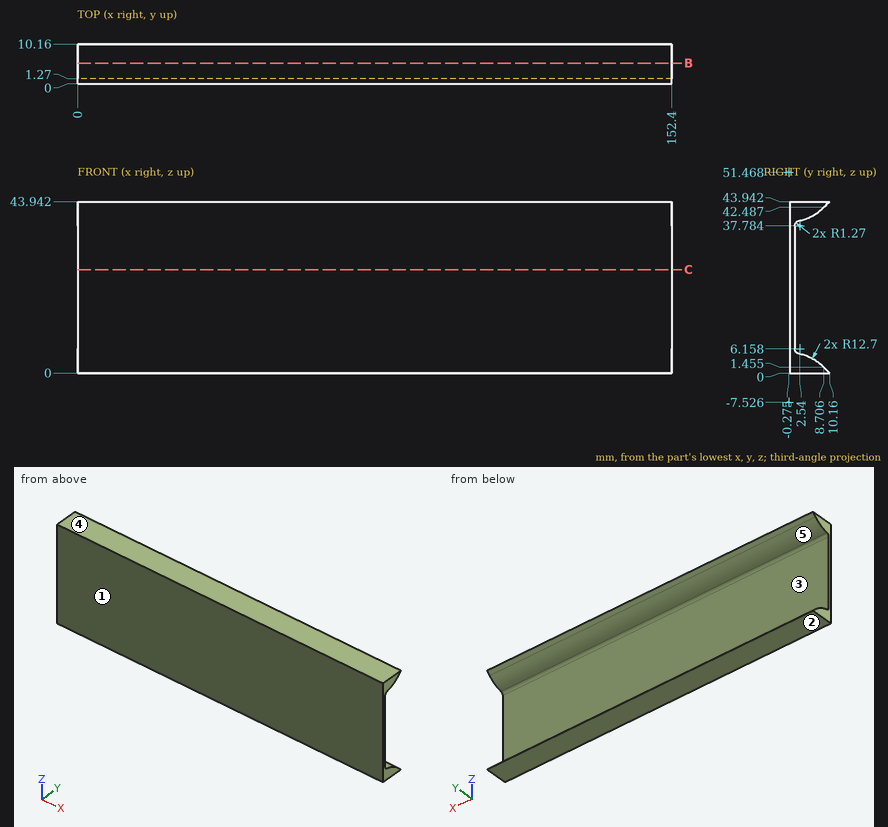
Geometry check sheet. Reference: drawing and pictorial views, mm from the part's lowest x, y, z. A direction names the side the tool comes from. Coordinates: 2 decimals unless noted, no trailing zeros. Order: outer loops, then holes, each group sorted by start corner. A loop starts at its lowest first (then second) coordinate and runs counter-clockwise, first axis right, second up. Notation, with made-up numbers: (-34.75, 31.5) -> (-22.75, 31.5) arc R30 ccw to (-22.75, 69.5) -> close; hole circle Ø5 at (4.5, -32). An arc over 180 degrees is marked (long way). Write item = value, one per line. Start each with the question number.
1) Go/stop test with flat-tipped pins: P1, Ø12, axis at x = 78, z = 27, coming from the +Y side; P2, Ø4, axis at y = 8.5, z = 5, coming from the -X side. Record where each tip stops, or that it passes through.
2) Mould release check, pull along Z, two halves, no side actions. Record for the marked faces 1, 2 and 3: +Z half, -Z half, draft (parallel to the pull), parting line (faces both ways), or undercut.
3) Cross-section at C-C (z = 26.5). Enter the section's corners in (x, y).
4) Material ranges on L1, parallel to Y at x = 13, z = 15; L2, parallel to Z at x = 111, y = 9; L3, parallel to Z at x = 10, y = 7 (1 decimal), recorded low to high.
5) Access from +Z, -Z, +X, -X, +Y, -Y to the whole of each face (thin tool, end or side, straight path). Record for the marked faces 4 and 5.
6) Cross-section at B-B (y = 5.25). Enter the section's corners in (x, z), then the cut area to 3 significant figures.
Ans:
q1.P1 = 1.27
q1.P2 = through
q2.face_1 = draft
q2.face_2 = -Z half
q2.face_3 = undercut
q3.outline = (0, 0) -> (152.4, 0) -> (152.4, 1.27) -> (0, 1.27) -> close
q4.L1 = 0 to 1.27
q4.L2 = 0 to 1.16, 42.78 to 43.94
q4.L3 = 0 to 2.9, 41.1 to 43.9
q5.face_4 = +Z, +X, -X, +Y, -Y
q5.face_5 = +X, -X, +Y
q6.outline = (0, 0) -> (152.4, 0) -> (152.4, 3.91) -> (0, 3.91) -> close; (0, 40.03) -> (152.4, 40.03) -> (152.4, 43.94) -> (0, 43.94) -> close
q6.area = 1,190 mm²
